Here's how the part is built. I have some questions about the finished solid (model axes, mm). Face numbers are marked on the shaded views. Give positions to 0.01 mm unless a question says otherwise; leave off trailing zeros. Order: outer loops, then holes, each group sorted by start corner. A loop starts at its lowest first (then second) coordinate and runs counter-clockwise, first axis right, second up. Notation, with made-up numbers: M 83.25,79.5 L 98.25,79.5 A15 ccw 98.25,108.5 Z; hole C 79,81.25 d3. An arc over 180 degrees is marked long. Use one line per item in the form item = value.
from build123d import *

# Parameters (mm, degrees)
SKETCH1_R          = 2
EXTRUDE1_DEPTH     = 1.6
SKETCH2_R          = 1
EXTRUDE2_DEPTH     = 6
CUT_EXTRUDE1_DEPTH = 0.5
FILLET1_R          = 0.2
CHAMFER1_SIZE      = 0.3
FILLET2_R          = 0.5


with BuildPart() as part:
    # Sketch1 → Extrude1 (new body)
    with BuildSketch(Plane.XY):
        Circle(SKETCH1_R)
    extrude(amount=EXTRUDE1_DEPTH)

    # Sketch2 → Extrude2 (add)
    with BuildSketch(Plane.XY.offset(1.6)):
        Circle(SKETCH2_R)
    extrude(amount=EXTRUDE2_DEPTH)

    # Sketch3 → Cut-Extrude1 (cut)
    with BuildSketch(Plane(origin=(0, 0, 0), x_dir=(-1, 0, 0), z_dir=(0, 0, -1))):
        Polygon((0.303448276, -0.280106101), (0.303448276, -1.258487543), (-0.331458886, -1.258487543), (-0.331458886, -0.280106101), (-1.343944387, -0.280106101), (-1.343944387, 0.382811671), (-0.331458886, 0.382811671), (-0.331458886, 1.389386448), (0.303448276, 1.389386448), (0.303448276, 0.382811671), (1.285259033, 0.382811671), (1.285259033, -0.280106101), align=None)
    extrude(amount=-CUT_EXTRUDE1_DEPTH, mode=Mode.SUBTRACT)

    # Fillet1
    fillet1_edges = [part.edges().sort_by_distance(p)[0] for p in [
        (0.331458886, 0.382811671, 0.25),
        (-0.303448276, 0.382811671, 0.25),
        (-0.303448276, -0.280106101, 0.25),
        (0.331458886, -0.280106101, 0.25),
    ]]
    fillet(fillet1_edges, radius=FILLET1_R)

    # Chamfer1
    chamfer1_edges = [part.edges().sort_by_distance(p)[0] for p in [
        (-1, 0, 7.6),
    ]]
    chamfer(chamfer1_edges, length=CHAMFER1_SIZE)

    # Fillet2
    fillet2_edges = [part.edges().sort_by_distance(p)[0] for p in [
        (-2, 0, 0),
    ]]
    fillet(fillet2_edges, radius=FILLET2_R)


solid = part.part
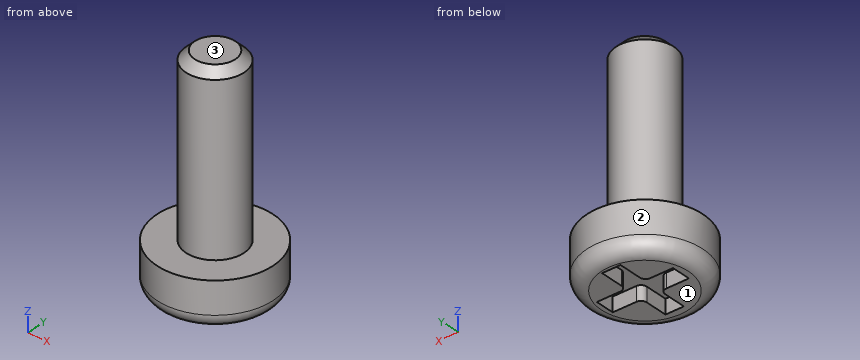
Q1. I'm going to push flat-ended pins straight in: pin 1 Ø1.5 at (x, z) = (-0.5, 3) entering from -Y; pin 2 Ø0.6 at (x, z) = (-0.5, 0.5) entering from -Y; pin 3 Ø0.6 at (x, z) = (1, 0) entering from +Y. Where does each tip first touch, or does it pass through?
Found:
pin_1 = -1
pin_2 = -1.99
pin_3 = 1.74
Q2. I want a section at B-B on x = 0. Write out the boundary of the cut face in (y, z), then the cut area to 3 significant figures.
Found:
outline = M -2,0.5 A0.5 ccw -1.5,0 L -1.26,0 L -1.26,0.5 L 1.39,0.5 L 1.39,0 L 1.5,0 A0.5 ccw 2,0.5 L 2,1.6 L 1,1.6 L 1,7.3 L 0.7,7.6 L -0.7,7.6 L -1,7.3 L -1,1.6 L -2,1.6 Z
area = 16.9 mm²
Q3. I want a section at C-C on z = 1. Write out the boundary of the cut face in (x, y).
Found:
outline = C 0,0 d4
Q4. I want a section at D-D on z = 2. Write out the boundary of the cut face in (x, y).
Found:
outline = C 0,0 d2
Q5. I need wall thicknesses on L1, parallel to Z at x = -0.9, y = 0.55; L2, parallel to X at y = -0.1, z = 1.25; L3, parallel to X at y = -1.25, z = 0.75. Which ranges of each line are inside material? Lowest first, please.
Found:
L1 = 0 to 1.6
L2 = -2 to 2
L3 = -1.56 to 1.56
Q6. I want a section at A-A on y = 0. Write out the boundary of the cut face in (x, z), then the cut area to 3 significant figures.
Found:
outline = M -2,0.5 A0.5 ccw -1.5,0 L -1.29,0 L -1.29,0.5 L 1.34,0.5 L 1.34,0 L 1.5,0 A0.5 ccw 2,0.5 L 2,1.6 L 1,1.6 L 1,7.3 L 0.7,7.6 L -0.7,7.6 L -1,7.3 L -1,1.6 L -2,1.6 Z
area = 16.9 mm²
Q7. Thinking about a two-plate mould opening in Z: for the marked faces 1, 2 and 3, which applies, +Z half, -Z half, draft (parallel to the pull), parting line (faces both ways), or undercut?
Found:
face_1 = -Z half
face_2 = draft
face_3 = +Z half
